Part model, mm, in its own coordinate system. Face numbers are marked on the shaded views. A direction names the side the tool comes from. Give positions to 0.01 mm unless a question says otherwise; leave off trailing zeros. Write each loop counter-clockwise with the first axis right and the second up, starting at its lowest first coordinate (ties: lowest second). Pieces come first, ordered by that corner, then holes.
Autodesk Inventor part; units mm, degrees
ref_plane "YZ Plane" through (0, 0, 0) normal (1, 0, 0) x (0, 1, 0)
ref_plane "XZ Plane" through (0, 0, 0) normal (0, 1, 0) x (-1, 0, 0)
ref_plane "XY Plane" through (0, 0, 0) normal (0, 0, 1) x (1, 0, 0)
sketch "草图1" plane through (0, 0, 0) normal (0, 1, 0) x (-1, 0, 0)
  circle A0 centre (0, 0) radius 12.5
  dimension "d0" = 25
extrude "拉伸1" add sketch "草图1" along normal blind 41
sketch "草图2" plane through (0, 41, 0) normal (0, 1, 0) x (1, 0, 0)
  circle A0 centre (0, 0) radius 3.5
  dimension "d3" = 7
extrude "拉伸2" add sketch "草图2" along normal blind 3
sketch "草图3" plane through (0, 44, 0) normal (0, 1, 0) x (1, 0, 0)
  circle A0 centre (0, 0) radius 2
  dimension "d6" = 4
extrude "拉伸3" add sketch "草图3" along normal blind 11
sketch "草图4" plane through (0, 55, 0) normal (0, 1, 0) x (1, 0, 0)
  line L0 (-4.637, -0.8) -> (5.5705, -0.8)
  line L1 (-17.5, 0) -> (17.5, 0)
  arc A0 (-1.833, -0.8) -> (1.833, -0.8) centre (0, 0) ccw
  dimension "d9" = 0.8
  dimension "d10" = 2
extrude "拉伸4" cut sketch "草图4" against normal blind 11
properties part number "电机" material "金色"
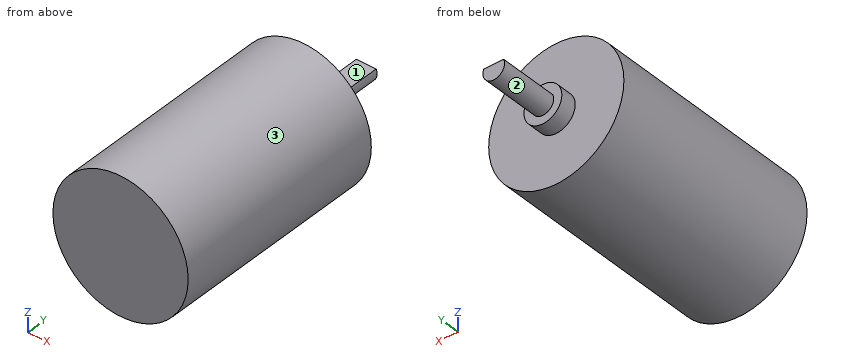
1) Wall check: L1, parallel to Y at x = -1.75, z = -9; L2, parallel to X at y = 3, z = 7.25; L3, parallel to Z at x = -7, y = 9. Give the ranges that are in metal, low to high.
Answers follow:
L1: y = 0 to 41
L2: x = -10.18 to 10.18
L3: z = -10.36 to 10.36
2) 3-axis set-ups, long thin cutter, end or side, ignore diameter. For the marked faces 1, 2 and 3: which of +Z, -Z, +X, -X, +Y, -Y reach the whole face in a straight line?
Answers follow:
face 1: +Z, +X, -X, +Y
face 2: +Y
face 3: +Y, -Y
3) Pin check, flat tips, straight feed: pin 1 Ø12 at (y, z) = (37.5, -9) entering from +X; pin 2 Ø2 at (y, z) = (38.5, -6) entering from -X; pin 3 Ø10 at (x, y) = (8.5, 8.5) entering from +Z. Stop position of each tip, or through.
Answers follow:
pin 1: stops at x = 12.13
pin 2: stops at x = -11.46
pin 3: stops at z = 12
4) Saw through at C-C, the plane y = 28. Write the cut outline in (x, z).
Answers follow:
outline: circle Ø25 at (0, 0)
5) Saw through at A-A, the plane z = 0. Write the cut outline in (x, y), then the cut area to 3 significant figures.
Answers follow:
outline: (-12.5, 0) - (12.5, 0) - (12.5, 41) - (3.5, 41) - (3.5, 44) - (2, 44) - (2, 55) - (-2, 55) - (-2, 44) - (-3.5, 44) - (-3.5, 41) - (-12.5, 41) - close
area: 1,090 mm2
6) Saw through at B-B, the plane x = 0. Write the cut outline in (y, z).
Answers follow:
outline: (0, -12.5) - (41, -12.5) - (41, -3.5) - (44, -3.5) - (44, -2) - (55, -2) - (55, 0.8) - (44, 0.8) - (44, 3.5) - (41, 3.5) - (41, 12.5) - (0, 12.5) - close
7) Saw through at D-D, the plane x = 7.25. Write the cut outline in (y, z), then the cut area to 3 significant figures.
Answers follow:
outline: (0, -10.18) - (41, -10.18) - (41, 10.18) - (0, 10.18) - close
area: 835 mm2
